from build123d import *

# Parameters (mm, degrees)
AUFSATZ_LINEAR_AUSTRAGEN1_DEPTH             = 2
FORMSENKUNG_F_R_M4_SENKSCHRAUBE_MIT_2_COUNT = 2
FORMSENKUNG_F_R_M4_SENKSCHRAUBE_MIT_2_PITCH = 470
SKIZZE5_W                                   = 500
SKIZZE5_H                                   = 8
SCHLITZ_OBEN_DEPTH                          = 10


with BuildPart() as part:
    # Skizze1 → Aufsatz-Linear austragen1 (new body)
    with BuildSketch(Plane.XY):
        Polygon((-339.903846154, 3), (160.096153846, 3), (160.096153846, -63), (130.095509739, -63), (130.095509739, -71), (-309.903846154, -71), (-309.903846154, -63), (-339.903846154, -63), align=None)
    extrude(amount=AUFSATZ_LINEAR_AUSTRAGEN1_DEPTH)

    # Skizze3 → Formsenkung für M4 Senkschraube mit Innensechskant1 (revolve, cut)
    with BuildSketch(Plane(origin=(145.096153846, -30, 2), x_dir=(0, -1, 0), z_dir=(1, 0, 0))):
        Polygon((0, 0), (0, 2), (2.4, 2), (2.4, 1.9), (4.3, 0), align=None)
    formsenkung_f_r_m4_senkschraube_mit_inne = revolve(axis=Axis((145.096153846, -30, 8.35), (0, 0, -1)), mode=Mode.SUBTRACT)

    # Formsenkung f_r M4 Senkschraube mit  2: Formsenkung für M4 Senkschraube mit Innensechskant1 ×2
    with Locations(*[(-i * FORMSENKUNG_F_R_M4_SENKSCHRAUBE_MIT_2_PITCH, 0, 0) for i in range(1, FORMSENKUNG_F_R_M4_SENKSCHRAUBE_MIT_2_COUNT)]):
        add(formsenkung_f_r_m4_senkschraube_mit_inne, mode=Mode.SUBTRACT)

    # Skizze5 → Schlitz Oben (cut)
    with BuildSketch(Plane(origin=(0, 0, 0), x_dir=(-1, 0, 0), z_dir=(0, 0, -1))):
        with Locations((89.903846154, -67)):
            Rectangle(SKIZZE5_W, SKIZZE5_H)
    extrude(amount=-SCHLITZ_OBEN_DEPTH, mode=Mode.SUBTRACT)


solid = part.part
Geometry check sheet. Reference: the model listing, model coordinates, mm. Round coordinates to 2 decimals unless told otherwise and drop trailing zeros. Answer in a Markdown table with one row per item.
(1) Draft check along Y on faces 1 (the face through (-86, -30, 0)), 2 (the face through (-326.606, -28.143, 0.219)). Enter one of: released by +Y, released by -Y, zero draft, split by the parting line, or undercut.
Responses:
| item | result |
|---|---|
| face 1 | zero draft |
| face 2 | undercut |
(2) Scan lines: probe 1 along X at (y, z) = (-30, 0.1); probe 2 along X at (y, z) = (-27.5, 1.1). Record each from-to range of solid material in increasing order. Write a range as from..to.
Responses:
| item | result |
|---|---|
| probe 1 | x = -339.9..-327.3, -322.5..142.7, 147.5..160.1 |
| probe 2 | x = -339.9..-327.21, -322.6..142.79, 147.4..160.1 |
(3) Go/stop test with a flat-tipped pin: P1, Ø4, axis at x = 145.1, y = -30, coming from the +Z side. Record where the tip stops, or that it passes through.
Responses:
| item | result |
|---|---|
| P1 | passes through |
